Could you check a few things on this drawing? It's one solid part, dimensions in mm from its lowest x, y, z. Give positions to 0.01 mm unless a question says otherwise; leave off trailing zeros. Loops run counter-clockwise (first coordinate to the right, second up) from the corner with the lowest first, then second, coordinate; pieces in that order, holes last.
1. Imagine slicing it at C-C (x = 0.75). List the corners of the cut face in (y, z) for me.
2. I need wall thicknesses on line 1 along Y through (x, z) = (0.2, 27.5); line 2 along Z through (x, y) = (0.5, 5.25); line 3 along Y through (x, z) = (0.9, 56). Which ranges of each line are inside material? Lowest first, please.
3. Imagine slicing it at A-A (z = 45). List the corners of the cut face in (x, y) for me, plus the area to 3 significant figures.
4. For P1, Ø1, axis at y = 5.5, z = 39, coming from the -X side, with a flat end and sliding along its axis, tell me the tip position at first contact or that it passes through.
5. Imagine slicing it at B-B (y = 5). List the corners of the cut face in (x, z) for me, plus the area to 3 significant figures.
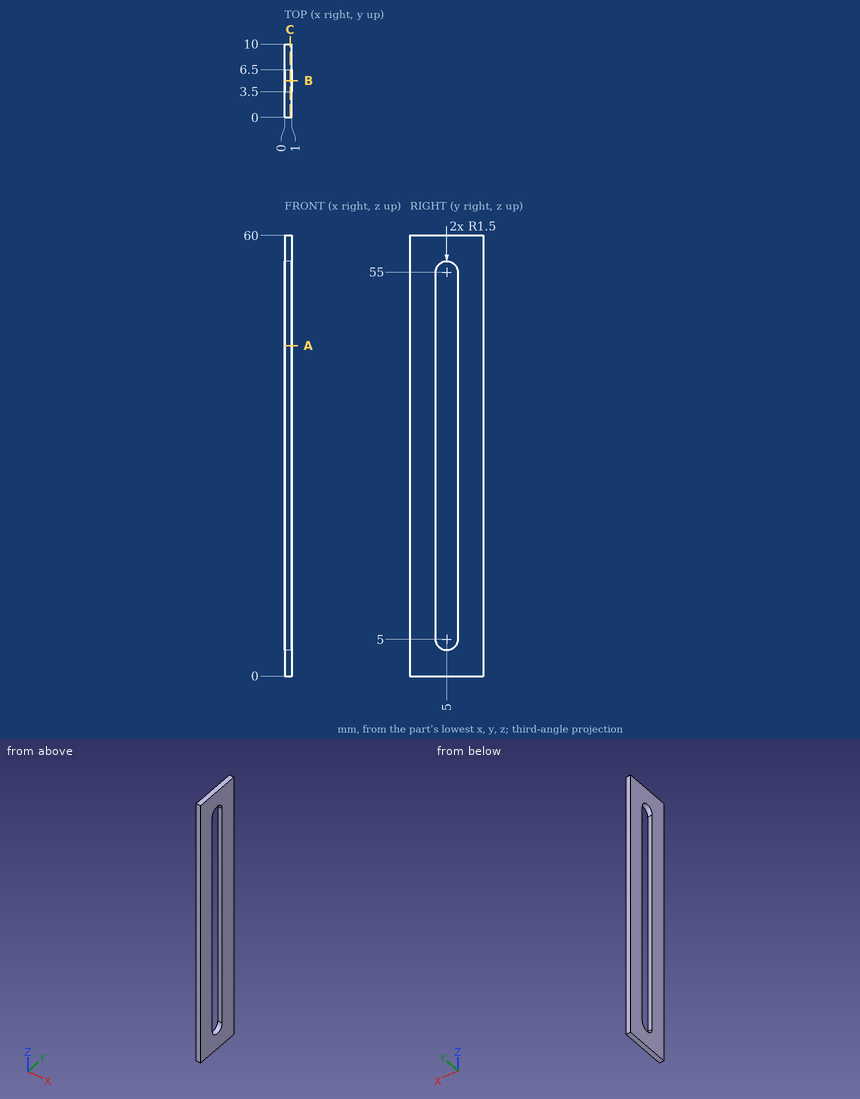
Derived:
1. outline: (0, 0) - (10, 0) - (10, 60) - (0, 60) - close; hole (3.5, 5) arc R1.5 ccw to (6.5, 5) - (6.5, 55) arc R1.5 ccw to (3.5, 55) - close
2. line 1: y = 0 to 3.5, 6.5 to 10
2. line 2: z = 0 to 3.52, 56.48 to 60
2. line 3: y = 0 to 3.88, 6.12 to 10
3. outline: (0, 0) - (1, 0) - (1, 3.5) - (0, 3.5) - close; (0, 6.5) - (1, 6.5) - (1, 10) - (0, 10) - close
3. area: 7.00 mm2
4. P1: passes through
5. outline: (0, 0) - (1, 0) - (1, 3.5) - (0, 3.5) - close; (0, 56.5) - (1, 56.5) - (1, 60) - (0, 60) - close
5. area: 7.00 mm2
